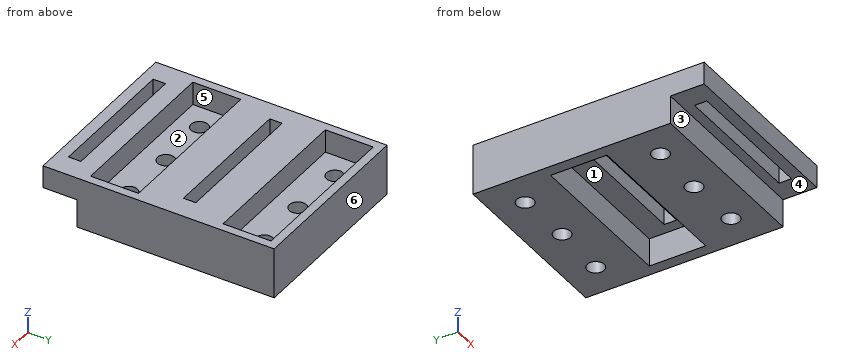
from build123d import *

# Parameters (mm, degrees)
SKETCH4_W                 = 32
SKETCH4_H                 = 35
BOSS_EXTRUDE1_DEPTH       = 9
SHELL1_T                  = -1.5
SHELL1_THICKNESS_2_FACE_W = 29
SHELL1_THICKNESS_2_FACE_H = 32
SHELL1_THICKNESS_2_DEPTH  = 3.4
SKETCH5_R                 = 1.5
CUT_EXTRUDE2_DEPTH        = 9
RIB6_REACH                = 27.362
SKETCH12_WALLS_W          = 81.724747412
SKETCH12_WALLS_H          = 15
SKETCH13_W                = 28
SKETCH13_H                = 10
CUT_EXTRUDE3_DEPTH        = 5
SKETCH15_W                = 24.5
SKETCH15_H                = 2.2
CUT_EXTRUDE4_DEPTH        = 10
SKETCH16_W                = 32
SKETCH16_H                = 4
BOSS_EXTRUDE2_DEPTH       = 6
SKETCH17_W                = 24
SKETCH17_H                = 2.2
CUT_EXTRUDE5_DEPTH        = 10


with BuildPart() as part:
    # Sketch4 → Boss-Extrude1 (new body)
    with BuildSketch(Plane.XY):
        Rectangle(SKETCH4_W, SKETCH4_H)
    extrude(amount=BOSS_EXTRUDE1_DEPTH)

    # Shell1
    shell1_openings = [part.faces().sort_by_distance(p)[0] for p in [
        (0, 0, 9),
    ]]
    offset(amount=SHELL1_T, openings=shell1_openings, kind=Kind.INTERSECTION)

    # Shell1 thickness 2 face (on inner face of the shell) → Shell1 thickness 2 (add)
    with BuildSketch(Plane(origin=(0, 0, 1.5), x_dir=(-1, 0, 0), z_dir=(0, 0, -1))):
        Rectangle(SHELL1_THICKNESS_2_FACE_W, SHELL1_THICKNESS_2_FACE_H)
    extrude(amount=-SHELL1_THICKNESS_2_DEPTH)

    # Sketch5 → Cut-Extrude2 (cut)
    with BuildSketch(Plane.XY.offset(4.9)):
        with Locations((-10, -12)):
            Circle(SKETCH5_R)
        with Locations((10, -12)):
            Circle(SKETCH5_R)
        with Locations((0, 11.7)):
            Circle(SKETCH5_R)
        with Locations((0, -11.7)):
            Circle(SKETCH5_R)
        with Locations((-10, 12)):
            Circle(SKETCH5_R)
        with Locations((10, 12)):
            Circle(SKETCH5_R)
    extrude(amount=-CUT_EXTRUDE2_DEPTH, mode=Mode.SUBTRACT)

    # Sketch12 walls → Rib6 (add, up to next)
    with BuildSketch(Plane.XY.offset(9), mode=Mode.PRIVATE) as rib6_sk1:
        Rectangle(SKETCH12_WALLS_W, SKETCH12_WALLS_H)
    rib6_tool1 = extrude(rib6_sk1.sketch, amount=-RIB6_REACH, mode=Mode.PRIVATE) - part.part
    add(rib6_tool1.solids().sort_by_distance((0, 0, 9))[0])

    # Sketch13 → Cut-Extrude3 (cut)
    with BuildSketch(Plane(origin=(0, 0, 0), x_dir=(-1, 0, 0), z_dir=(0, 0, -1))):
        Rectangle(SKETCH13_W, SKETCH13_H)
    extrude(amount=-CUT_EXTRUDE3_DEPTH, mode=Mode.SUBTRACT)

    # Sketch15 → Cut-Extrude4 (cut)
    with BuildSketch(Plane(origin=(0, 0, 5), x_dir=(-1, 0, 0), z_dir=(0, 0, -1))):
        with Locations((0.25, 0)):
            Rectangle(SKETCH15_W, SKETCH15_H)
    extrude(amount=-CUT_EXTRUDE4_DEPTH, mode=Mode.SUBTRACT)

    # Sketch16 → Boss-Extrude2 (add)
    with BuildSketch(Plane.XZ.offset(17.5)):
        with Locations((0, 7)):
            Rectangle(SKETCH16_W, SKETCH16_H)
    extrude(amount=BOSS_EXTRUDE2_DEPTH)

    # Sketch17 → Cut-Extrude5 (cut)
    with BuildSketch(Plane.XY.offset(9)):
        with Locations((0, -20.38)):
            Rectangle(SKETCH17_W, SKETCH17_H)
    extrude(amount=-CUT_EXTRUDE5_DEPTH, mode=Mode.SUBTRACT)


solid = part.part
Geometry check sheet. Reference: the model listing, model coordinates, mm. Face numbers are marked on the shaded views. A direction names the side the tool comes from. Round coordinates to 2 decimals unless told otherwise and drop trailing zeros. Loops run counter-clockwise (first coordinate to the right, second up) from the corner with the lowest first, then second, coordinate; pieces in that order, holes last. Notation, with made-up numbers: (50.5, 59.5) -> (109.5, 59.5) arc R25 ccw to (109.5, 86.5) -> close; hole circle Ø5 at (10.5, 78.5). An arc over 180 degrees is marked (long way). Answer as a JSON object with one key per item and string values. Group by question number.
Item 1: Cross-section at B-B, the plane z = 8. Record the cut outline in (x, y), plus the area to 3 significant figures.
Item 2: Thickness scan on line 1 along Y through (x, z) = (-10, 1.8); line 2 along Y through (x, z) = (0, 3.8); line 3 along Y through (x, z) = (4.5, 6). Record the ranges inside material, lowest first.
Item 3: Set-up check for the marked faces 1, 2 and 3: record each of +Z, -Z, +X, -X, +Y, -Y from which the full face is reachable in a straight line by a thin tool's end or side.
Item 4: Cross-section at A-A, the plane x = -5. Record the cut outline in (y, z).
Item 5: Depth check by flat-ended pin: pin 1 Ø7 at (x, y) = (-3.5, 12) entering from +Z; pin 2 Ø5 at (x, y) = (-5, -1) entering from -Z; pin 3 Ø1.8 at (x, y) = (-10, -12) entering from +Z. Enter the tip coordinate at first touch or a pass-through.
Item 6: Cross-section at D-D, the plane x = -10. Count the separate pieces of the cut face and the enclosed holes in it, plus the area to 3 significant figures.
Item 7: Release check for a two-part mould opening along Y. For the marked faces 4, 5 and 6 record: pulls with the +Y half, pulls with the -Y half, needs draft (parallel to the pull), parting line crosses it, or undercut.
Item 8: Cross-section at C-C, the plane y = 8. Record the cut outline in (x, z).
Determined:
{
 "1": {"outline": "(-16, -23.5) -> (16, -23.5) -> (16, 17.5) -> (-16, 17.5) -> close; hole (-14.5, -16) -> (14.5, -16) -> (14.5, -7.5) -> (-14.5, -7.5) -> close; hole (-14.5, 7.5) -> (14.5, 7.5) -> (14.5, 16) -> (-14.5, 16) -> close; hole (-12.5, -1.1) -> (12, -1.1) -> (12, 1.1) -> (-12.5, 1.1) -> close; hole (-12, -21.48) -> (12, -21.48) -> (12, -19.28) -> (-12, -19.28) -> close", "area": "712 mm²"},
 "2": {"line 1": "y = -17.5 to -13.5, -10.5 to -5, 5 to 10.5, 13.5 to 17.5", "line 2": "y = -17.5 to -13.2, -10.2 to -5, 5 to 10.2, 13.2 to 17.5", "line 3": "y = -23.5 to -21.48, -19.28 to -16, -7.5 to -1.1, 1.1 to 7.5, 16 to 17.5"},
 "3": {"face 1": "-Z", "face 2": "+Z", "face 3": "-Z, +X, -X, -Y"},
 "4": {"outline": "(-23.5, 5) -> (-21.48, 5) -> (-21.48, 9) -> (-23.5, 9) -> close; (-19.28, 5) -> (-17.5, 5) -> (-17.5, 0) -> (-5, 0) -> (-5, 5) -> (-1.1, 5) -> (-1.1, 9) -> (-7.5, 9) -> (-7.5, 4.9) -> (-16, 4.9) -> (-16, 9) -> (-19.28, 9) -> close; (1.1, 5) -> (5, 5) -> (5, 0) -> (17.5, 0) -> (17.5, 9) -> (16, 9) -> (16, 4.9) -> (7.5, 4.9) -> (7.5, 9) -> (1.1, 9) -> close"},
 "5": {"pin 1": "stops at z = 4.9", "pin 2": "stops at z = 5", "pin 3": "passes through"},
 "6": {"separate pieces": "5", "enclosed holes": "0", "area": "172 mm²"},
 "7": {"face 4": "needs draft", "face 5": "undercut", "face 6": "pulls with the +Y half"},
 "8": {"outline": "(-16, 0) -> (16, 0) -> (16, 9) -> (14.5, 9) -> (14.5, 4.9) -> (-14.5, 4.9) -> (-14.5, 9) -> (-16, 9) -> close"}
}
